```python
from build123d import *

# Parameters (mm, degrees)
F0_W     = 50
F0_H     = 45
F0_W_2   = 13.365347
F0_H_2   = 12.623919
F0_R     = 1
F0_R_2   = 1.5
F0_R_3   = 5
F1_DEPTH = 3.5


with BuildPart() as f1:
    # F0 (on Top) → F1 (new body)
    with BuildSketch(Plane.XY):
        Rectangle(F0_W, F0_H)
        with Locations((-13.817327, -11.68804)):
            Rectangle(F0_W_2, F0_H_2, mode=Mode.SUBTRACT)
        with Locations((0, -17.25)):
            Circle(F0_R, mode=Mode.SUBTRACT)
        with Locations((-17.25, 0)):
            Circle(F0_R, mode=Mode.SUBTRACT)
        with Locations((-15, 15.75)):
            Circle(F0_R_2, mode=Mode.SUBTRACT)
        Circle(F0_R_3, mode=Mode.SUBTRACT)
        with Locations((17.25, 0)):
            Circle(F0_R, mode=Mode.SUBTRACT)
        with Locations((0, 17.25)):
            Circle(F0_R, mode=Mode.SUBTRACT)
        with Locations((15, 15.75)):
            Circle(F0_R_2, mode=Mode.SUBTRACT)
    extrude(amount=F1_DEPTH)


solid = f1.part
```
Can you work these out from the model? Positions are in its coordinate system, mm. A direction names the side the tool comes from. Round coordinates to 2 decimals unless told otherwise and drop trailing zeros. Loops run counter-clockwise (first coordinate to the right, second up) from the corner with the lowest first, then second, coordinate; pieces in that order, holes last. Notation, with made-up numbers: M 73,75 L 131,75 A29 ccw 131,100 Z; hole C 20,-8 d4. An arc over 180 degrees is marked long. Answer in a Markdown table with one row per item.
1. If we section it at C-C, the plane z = 2.8: Give the number of separate pieces and of enclosed holes in the cut face, plus the area to 3 significant figures.
Established:
| item | result |
|---|---|
| separate pieces | 1 |
| enclosed holes | 8 |
| area | 1,980 mm² |
2. If we section it at B-B, the plane x = -15: Please give me the cut outline in (y, z).
Established:
| item | result |
|---|---|
| outline | M -22.5,0 L -18,0 L -18,3.5 L -22.5,3.5 Z; M -5.38,0 L 14.25,0 L 14.25,3.5 L -5.38,3.5 Z; M 17.25,0 L 22.5,0 L 22.5,3.5 L 17.25,3.5 Z |
3. If we section it at A-A, the plane y = -15.5: Please give me the cut outline in (x, z), plus the area to 3 significant figures.
Established:
| item | result |
|---|---|
| outline | M -25,0 L -20.5,0 L -20.5,3.5 L -25,3.5 Z; M -7.13,0 L 25,0 L 25,3.5 L -7.13,3.5 Z |
| area | 128 mm² |
4. On a 3-axis mill with a long thin cutter (end or side, diameter ignored), from which of +Z, -Z, +X, -X, +Y, -Y can I reach the whole of each face in a straight line? I mean faces 4 (the face through (25, 0, 2)), 5 (the face through (-20.5, -12, 2)). Say none if no direction works.
Established:
| item | result |
|---|---|
| face 4 | +Z, -Z, +X, +Y, -Y |
| face 5 | +Z, -Z |
5. If we section it at D-D, the plane x = 17.25: Please give me the cut outline in (y, z), plus the area to 4 significant figures.
Established:
| item | result |
|---|---|
| outline | M -22.5,0 L -1,0 L -1,3.5 L -22.5,3.5 Z; M 1,0 L 22.5,0 L 22.5,3.5 L 1,3.5 Z |
| area | 150.5 mm² |
6. I'm going to push a flat-ended pin straight in: pin 1 Ø9 at (x, y) = (0, 0) entering from -Z. Where does the tip first touch, or does it pass through?
Established:
| item | result |
|---|---|
| pin 1 | through |
7. Thinking about a two-plate mould opening in X: for faces 1 (the face through (-16.326, -0.383, 1.726)), 2 (the face through (-25, 0, 2)), 3 (the face through (0, -22.5, 2)), which applies, pulls with the +X half, pulls with the -X half, needs draft (parallel to the pull), parting line crosses it, or undercut?
Established:
| item | result |
|---|---|
| face 1 | undercut |
| face 2 | pulls with the -X half |
| face 3 | needs draft |
8. Please list where these lines run through material, in increasing order: line 1 (Y direction, x = -15, z = 1.75); line 2 (Y direction, x = 0, z = 2.75); line 3 (X direction, y = -16, z = 1.2). Write a range as from..to.
Established:
| item | result |
|---|---|
| line 1 | -22.5..-18, -5.38..14.25, 17.25..22.5 |
| line 2 | -22.5..-18.25, -16.25..-5, 5..16.25, 18.25..22.5 |
| line 3 | -25..-20.5, -7.13..25 |
